Design review of the part built by this model. Coordinates are the model's own, in mm. Face numbers are marked on the shaded views. Coordinates: 2 decimals unless noted, no trailing zeros. Write each loop counter-clockwise with the first axis right and the second up, starting at its lowest first coordinate (ties: lowest second). Pieces come first, ordered by that corner, then holes. Notation, with made-up numbers: (-9, 77.5) - (5, 77.5) arc R6 ccw to (5, 84.5) - close; hole circle Ø8 at (-13, -21.75). An arc over 180 degrees is marked (long way). One line per item, written item: value.
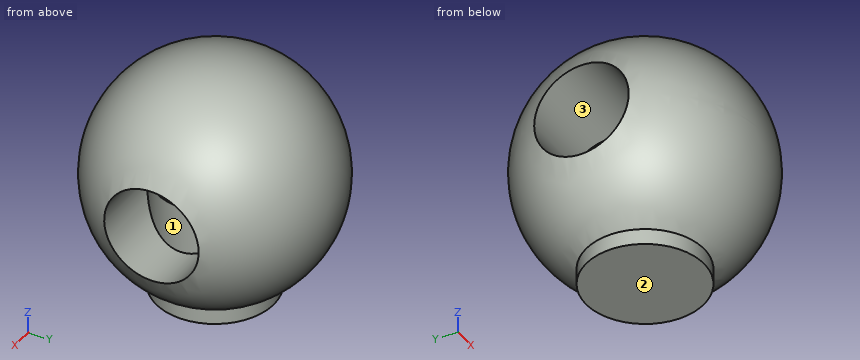
Autodesk Inventor part; units mm, degrees
ref_plane "XY Plane" through (0, 0, 0) normal (0, 0, 1) x (1, 0, 0)
sketch "スケッチ1" plane through (0, 0, 0) normal (0, 0, 1) x (1, 0, 0)
  arc A0 (0, 50) -> (0, -50) centre (0, 0) ccw
  line L0 (0, 50) -> (0, -50)
  dimension "d0" = 100
revolve "回転1" add sketch "スケッチ1" angle 360 about axis through (0, 50, 0) along (0, -1, 0)
sketch "スケッチ3" plane through (0, 0, 0) normal (1, 0, 0) x (0, 1, 0)
  circle A0 centre (0, 0) radius 20
  dimension "d4" = 40
extrude "押し出し2" cut sketch "スケッチ3" along normal mid plane 100
sketch "スケッチ4" plane through (0, 0, 0) normal (0, 0, 1) x (1, 0, 0)
  circle A0 centre (0, 0) radius 25
  dimension "d7" = 50
extrude "押し出し3" add sketch "スケッチ4" against normal blind 50
properties part number "UpperlegR"
1. Insertion check: pin 1 Ø1.5 at (y, z) = (-24, 10.5) entering from +X; pin 2 Ø2 at (x, z) = (13, 26.5) entering from -Y; pin 3 Ø10 at (x, y) = (-8, -16) entering from +Z. Each pin has a flat end and moves straight along its axis. Give the tip position at first contact, or say it passes through.
Answer block:
pin 1: stops at x = 43.04
pin 2: stops at y = -41.07
pin 3: stops at z = 48.31
2. Mouldability with a two-part tool opening along Y and no side actions: class the marked faces 1, 2 and 3 as released by +Y, released by -Y, zero draft, split by the parting line, or undercut.
Answer block:
face 1: undercut
face 2: zero draft
face 3: undercut
3. Consider section D-D, the plane x = 12. Write out the cut boundary in (y, z), then the cut area to 3 significant figures.
Answer block:
outline: (-21.93, -50) - (21.93, -50) - (21.93, -43.3) arc R48.54 ccw (long way) to (-21.93, -43.3) - close; hole (-20, 0) - (20, 0) arc R20 ccw to start
area: 6,910 mm^2
4. Wall thickness on line 1 along Z through (x, y) = (-4, 0); line 2 along Z through (x, y) = (-8, 0); line 3 along X through (y, z) = (43, -15): over which ranges is each line inside the solid? List them lowest first.
Answer block:
line 1: z = -50 to 0, 20 to 49.84
line 2: z = -50 to 0, 20 to 49.36
line 3: x = -20.64 to 20.64
5. Consider section B-B, the plane x = 0. Write out the cut boundary in (y, z).
Answer block:
outline: (-25, -50) - (25, -50) - (25, -43.3) arc R50 ccw (long way) to (-25, -43.3) - close; hole (-20, 0) - (20, 0) arc R20 ccw to start
6. Consider section C-C, the plane z = -12.5. Write out the cut boundary in (x, y), then the cut area to 3 significant figures.
Answer block:
outline: (-45.83, -15.61) arc R48.41 ccw to (45.83, -15.61) - (19.53, -15.61) arc R25 ccw to (19.53, 15.61) - (45.83, 15.61) arc R48.41 ccw to (-45.83, 15.61) - (-19.53, 15.61) arc R25 ccw to (-19.53, -15.61) - close
area: 5,850 mm^2
7. Consider section A-A, the plane y = 0. Write out the cut boundary in (x, z).
Answer block:
outline: (-45.83, -20) arc R50 ccw to (-25, -43.3) - (-25, -50) - (25, -50) - (25, -43.3) arc R50 ccw to (45.83, -20) - (25, -20) - (25, 0) - (-25, 0) - (-25, -20) - close; (-45.83, 20) - (45.83, 20) arc R50 ccw to start
